Build history of the part. All positions in model axes, mm. Face numbers are marked on the shaded views. A direction names the side the tool comes from. Coordinates: 2 decimals unless noted, no trailing zeros. Order: outer loops, then holes, each group sorted by start corner. A loop starts at its lowest first (then second) coordinate and runs counter-clockwise, first axis right, second up. Notation, with made-up numbers: (6, 5.5) -> (53, 5.5) arc R21 ccw to (53, 31.5) -> close; hole circle Ø11 at (-31.5, -6.75). An arc over 180 degrees is marked (long way). Write each question's results on one line, items separated by ' | '.
from build123d import *

# Parameters (mm, degrees)
BOSS_EXTRUDE2_DEPTH = 100
SKETCH2_R           = 2.5
SKETCH2_R_2         = 3
CUT_EXTRUDE1_DEPTH  = 10
SKETCH3_R           = 2.5
CUT_EXTRUDE2_DEPTH  = 10
SKETCH4_R           = 2
CUT_EXTRUDE3_DEPTH  = 10
SKETCH5_W           = 40
SKETCH5_H           = 20
CUT_EXTRUDE4_DEPTH  = 163.249807396
SKETCH6_W           = 5
SKETCH6_H           = 12
BOSS_EXTRUDE3_DEPTH = 15
BOSS_EXTRUDE4_DEPTH = 5
SKETCH9_R           = 3
CUT_EXTRUDE5_DEPTH  = 7
BOSS_EXTRUDE5_DEPTH = 1


with BuildPart() as part:
    # Sketch1 → Boss-Extrude2 (new body)
    with BuildSketch(Plane.XY):
        Polygon((-50, 5), (50, 5), (50, 65), (55, 65), (55, 0), (-55, 0), (-55, 65), (-50, 65), align=None)
    extrude(amount=BOSS_EXTRUDE2_DEPTH)

    # Sketch2 → Cut-Extrude1 (cut)
    with BuildSketch(Plane(origin=(0, 5, 0), x_dir=(1, 0, 0), z_dir=(0, 1, 0))):
        with Locations(Location((0, -50, 0), (0, 0, 270))):
            Circle(SKETCH2_R)
        with Locations(Location((0, -30, 0), (0, 0, 180))):
            Circle(SKETCH2_R_2)
    extrude(amount=-CUT_EXTRUDE1_DEPTH, mode=Mode.SUBTRACT)

    # Sketch3 → Cut-Extrude2 (cut)
    with BuildSketch(Plane.ZY.offset(55)):
        with Locations((80, 20)):
            Circle(SKETCH3_R)
        with Locations((20, 55)):
            Circle(SKETCH3_R)
    extrude(amount=-CUT_EXTRUDE2_DEPTH, mode=Mode.SUBTRACT)

    # Sketch4 → Cut-Extrude3 (cut)
    with BuildSketch(Plane(origin=(55, 0, 0), x_dir=(0, 0, -1), z_dir=(1, 0, 0))):
        with Locations((-80, 15)):
            Circle(SKETCH4_R)
    extrude(amount=-CUT_EXTRUDE3_DEPTH, mode=Mode.SUBTRACT)

    # Sketch5 → Cut-Extrude4 (cut, through all)
    with BuildSketch(Plane.ZY.offset(55)):
        with Locations((70, 20)):
            Rectangle(SKETCH5_W, SKETCH5_H)
    extrude(amount=-CUT_EXTRUDE4_DEPTH, mode=Mode.SUBTRACT)

    # Sketch6 → Boss-Extrude3 (add)
    with BuildSketch(Plane(origin=(0, 5, 0), x_dir=(1, 0, 0), z_dir=(0, 1, 0))):
        with Locations((13.5, -80)):
            Rectangle(SKETCH6_W, SKETCH6_H)
    extrude(amount=BOSS_EXTRUDE3_DEPTH)

    # Sketch8 → Boss-Extrude4 (add)
    with BuildSketch(Plane.ZY.offset(-11)):
        with BuildLine():
            Line((74, 20), (86, 20))
            ThreePointArc((86, 20), (80, 26), (74, 20))
        make_face()
    extrude(amount=-BOSS_EXTRUDE4_DEPTH)

    # Sketch9 → Cut-Extrude5 (cut)
    with BuildSketch(Plane.ZY.offset(-11)):
        with Locations((80, 20)):
            Circle(SKETCH9_R)
    extrude(amount=-CUT_EXTRUDE5_DEPTH, mode=Mode.SUBTRACT)

    # Sketch10 → Boss-Extrude5 (add)
    with BuildSketch(Plane(origin=(0, 5, 0), x_dir=(1, 0, 0), z_dir=(0, 1, 0))):
        Polygon((14, -86.5), (16.5, -86.5), (16.5, -81.5), (16, -81.5), (16, -86), (14, -86), align=None)
    extrude(amount=BOSS_EXTRUDE5_DEPTH)


solid = part.part
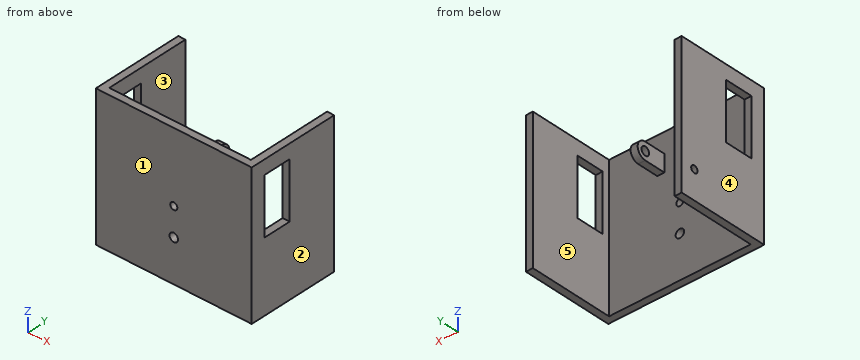
Item 1: Pull direction X, two halves, no side cores. Call the marked faces 1, 2 and 3: released by +X, released by -X, zero draft, split by the parting line, or undercut.
Answer:
face 1: zero draft | face 2: released by +X | face 3: undercut
Item 2: Slice it at C-C, the plane z = 20. List the corners of the cut face in (x, y).
Answer:
outline: (-55, 0) -> (55, 0) -> (55, 65) -> (50, 65) -> (50, 5) -> (-50, 5) -> (-50, 52.5) -> (-55, 52.5) -> close; (-55, 57.5) -> (-50, 57.5) -> (-50, 65) -> (-55, 65) -> close
Item 3: Slice it at B-B, the plane y = 37. List the corners of the cut face in (x, z), and give its area (3 significant figures).
Answer:
outline: (-55, 0) -> (-50, 0) -> (-50, 100) -> (-55, 100) -> close; (50, 0) -> (55, 0) -> (55, 100) -> (50, 100) -> close | area: 1,000 mm^2
Item 4: Slice it at D-D, the plane y = 55. List the corners of the cut face in (x, z), and give its area (3 significant figures).
Answer:
outline: (-55, 0) -> (-50, 0) -> (-50, 17.5) -> (-55, 17.5) -> close; (-55, 22.5) -> (-50, 22.5) -> (-50, 100) -> (-55, 100) -> close; (50, 0) -> (55, 0) -> (55, 100) -> (50, 100) -> close | area: 975 mm^2
Item 5: Drill centre lines: line 1 (X direction, y = 34.5, z = 6.5); line 2 (Y direction, x = -51.5, z = 20); line 3 (Y direction, x = 13.8, z = 80). Where is each one in solid material? Low to high. Write a range as from..to.
Answer:
line 1: x = -55..-50, 50..55 | line 2: y = 0..52.5, 57.5..65 | line 3: y = 0..17, 23..26
Item 6: Pin check, flat tips, straight feed: pin 1 (1.5 mm diameter, centred on x = -53, y = 25, fed in from -Z); pin 2 (1.5 mm diameter, centred on x = 12.5, y = 15, fed in from +Z); pin 3 (2 mm diameter, centred on x = 0, z = 41, fed in from +Y); pin 4 (0.8 mm diameter, centred on x = 16, y = 5.5, fed in from +Z). Stop position of each tip, or through.
Answer:
pin 1: stops at z = 0 | pin 2: stops at z = 86 | pin 3: stops at y = 5 | pin 4: stops at z = 86.5
Item 7: Tool access for the marked faces 4 and 5: list every direction of +Z, -Z, +X, -X, +Y, -Y with a clear straight run to the whole face (end or side of a thin tool).
Answer:
face 4: +Z, -Z, -X, +Y, -Y | face 5: +Z, -Z, +Y
Item 8: Slice it at A-A, the plane z = 80. List the corners of the cut face in (x, y).
Answer:
outline: (-55, 0) -> (55, 0) -> (55, 10) -> (50, 10) -> (50, 5) -> (16, 5) -> (16, 17) -> (11, 17) -> (11, 5) -> (-50, 5) -> (-50, 10) -> (-55, 10) -> close; (-55, 30) -> (-50, 30) -> (-50, 65) -> (-55, 65) -> close; (11, 23) -> (16, 23) -> (16, 26) -> (11, 26) -> close; (50, 30) -> (55, 30) -> (55, 65) -> (50, 65) -> close
